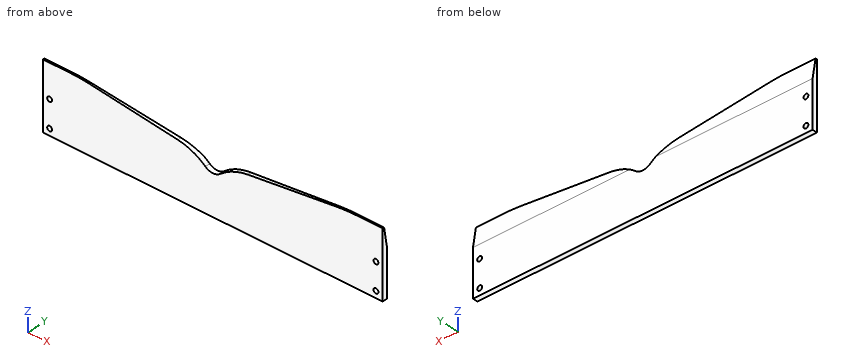
Autodesk Inventor part; units mm, degrees
ref_plane "YZ Plane" through (0, 0, 0) normal (1, 0, 0) x (0, 1, 0)
ref_plane "XZ Plane" through (0, 0, 0) normal (0, 1, 0) x (-1, 0, 0)
ref_plane "XY Plane" through (0, 0, 0) normal (0, 0, 1) x (1, 0, 0)
sketch "Sketch1" plane through (0, 0, 0) normal (0, 1, 0) x (-1, 0, 0)
  line L0 (0, 0) -> (-323.85, 0)
  line L1 (-323.85, 0) -> (-323.85, 63.5)
  line L2 (-323.85, 63.5) -> (0, 63.5)
  line L3 (0, 63.5) -> (0, 0)
  line L4 (-323.85, 0) -> (-323.85, 6.35)
  line L5 (0, 0) -> (-6.35, 0)
  line L6 (-323.85, 0) -> (-317.5, 0)
  line L7 (-323.85, 6.35) -> (-317.5, 6.35)
  line L8 (-317.5, 6.35) -> (-317.5, 31.75)
  line L9 (-6.35, 0) -> (-6.35, 6.35)
  line L10 (-6.35, 6.35) -> (-6.35, 31.75)
  circle A0 centre (-6.35, 6.35) radius 2.3241
  circle A1 centre (-6.35, 31.75) radius 2.3241
  circle A2 centre (-317.5, 31.75) radius 2.3241
  circle A3 centre (-317.5, 6.35) radius 2.3241
  line L11 (-161.925, 0) -> (-161.925, 38.1)
  line L12 (-161.925, 63.5) -> (-288.925, 63.5)
  line L13 (-161.925, 63.5) -> (-34.925, 63.5)
  line L14 (-161.925, 63.5) -> (-161.925, 38.1)
  line L15 (-161.925, 63.5) -> (-161.925, 57.15)
  circle A4 centre (-161.925, 63.5) radius 9.525
  circle A5 centre (-161.925, 49.2261) radius 11.1261
  line L16 (-288.925, 63.5) -> (-171.45, 43.4759)
  line L17 (-34.925, 63.5) -> (-152.4, 43.4759)
  line L18 (-288.925, 63.5) -> (-173.0511, 49.2261)
  line L19 (-34.925, 63.5) -> (-150.7989, 49.2261)
  dimension "d0" = 323.85
  dimension "d1" = 63.5
  dimension "d2" = 6.35
  dimension "d3" = 6.35
  dimension "d4" = 6.35
  dimension "d5" = 25.4
  dimension "d6" = 6.35
  dimension "d7" = 25.4
  dimension "d8" = 4.6482
  dimension "d9" = 4.6482
  dimension "d10" = 4.6482
  dimension "d11" = 4.6482
  dimension "d12" = 38.1
  dimension "d13" = 127
  dimension "d14" = 127
  dimension "d15" = 6.35
  dimension "d16" = 19.05
extrude "Extrusion1" add sketch "Sketch1" along normal blind 4.7625 contours L0 L11 A5 L17 L2 L3 | L0 L1 L2 L16 A5 L11
extrude "Extrusion2" add sketch "Sketch1" along normal blind 4.7625 contours L17 A5 L19 | L16 L18 A5
fillet "Fillet1" radius 50.8 2 edges at (173.0511, 2.3813, 49.2261) (150.7989, 2.3813, 49.2261)
fillet "Fillet2" radius 152.4 2 edges at (288.925, 2.3813, 63.5) (34.925, 2.3813, 63.5)
sketch "Sketch2" plane through (0, 0, 0) normal (-1, 0, 0) x (0, 0, 1)
  line L0 (63.5, 0) -> (63.5, 4.7625)
  line L1 (63.5, 0) -> (63.5, 1.5875)
  line L2 (63.5, 1.5875) -> (50.4087, 4.7625)
  line L3 (0, 4.7625) -> (63.5, 4.7625)
  line L4 (63.5, 4.7625) -> (50.4087, 4.7625)
  line L5 (63.5, 1.5875) -> (63.5, 4.7625)
  line L6 (63.5, 1.5875) -> (44.4761, 4.7625)
  line L7 (44.4761, 4.7625) -> (50.4087, 4.7625)
  point P0 (0, 0)
  dimension "d24" = 1.5875
extrude "Extrusion3" cut sketch "Sketch2" against normal through all
properties part number "lady brown aligner"
Read the model definition and answer for the solid it produces. Units are mm, in the model's axes. Round coordinates to 2 decimals unless told otherwise and drop trailing zeros. Write each loop counter-clockwise with the first axis right and the second up, starting at its lowest first coordinate (ties: lowest second). Pieces come first, ordered by that corner, then holes. Notation, with made-up numbers: (-21.75, -26.5) - (-16.75, -26.5) arc R13 cw to (-16.75, -1.5) - close; hole circle Ø7 at (-23.75, -7). An arc over 180 degrees is marked (long way). Use a Markdown table: item, result.
(1) The part is cut by section B-B (z = 47.5). Write down the section's boundary in (x, y).
Reported:
| item | result |
|---|---|
| outline | (0, 0) - (144.06, 0) - (144.06, 4.26) - (0, 4.26) - close; (179.79, 0) - (323.85, 0) - (323.85, 4.26) - (179.79, 4.26) - close |
(2) The part is cut by section D-D (x = 140). Write down the section's boundary in (y, z).
Reported:
| item | result |
|---|---|
| outline | (0, 0) - (4.76, 0) - (4.76, 44.48) - (3.97, 49.2) - (0, 49.2) - close |
(3) The part is cut by section C-C (x = 251). Write down the section's boundary in (y, z), then the cut area to 3 significant figures.
Reported:
| item | result |
|---|---|
| outline | (0, 0) - (4.76, 0) - (4.76, 44.48) - (2.37, 58.83) - (0, 58.83) - close |
| area | 263 mm2 |
(4) Straight lines are drawn through the part: line 1 along X through (y, z) = (0.85, 30); line 2 along Y through (x, z) = (307, 44.5); line 3 along Z through (x, y) = (148.5, 2.4). For each, find the intervals that lie inside material, in ascending order. Write a range as [from, to].
Reported:
| item | result |
|---|---|
| line 1 | [0, 4.82], [7.88, 315.97], [319.03, 323.85] |
| line 2 | [0, 4.76] |
| line 3 | [0, 45.13] |
(5) The part is cut by section A-A (y = 2.5). State how many separate pieces and enclosed holes the cut face has, then the cut area to 3 significant figures.
Reported:
| item | result |
|---|---|
| separate pieces | 1 |
| enclosed holes | 4 |
| area | 17,600 mm2 |
(6) Each of these flat-tipped pins is pushed along its axis until it touches: pin 1 Ø4 at (x, z) = (6.35, 31.75) entering from +Y; pin 2 Ø6 at (x, z) = (317.5, 31.75) entering from -Y; pin 3 Ø4 at (x, z) = (45, 54) entering from +Y; pin 4 Ø2 at (x, z) = (84.5, 57) entering from +Y. Where does it stop, or does it pass through?
Reported:
| item | result |
|---|---|
| pin 1 | through |
| pin 2 | y = 0 |
| pin 3 | y = 3.51 |
| pin 4 | y = 2.84 |
